```python
from build123d import *

# Parameters (mm, degrees)
F0_W     = 220
F0_H     = 25
F1_DEPTH = 15
F2_W     = 5
F2_H     = 25
F3_DEPTH = 225
F5_DEPTH = 25
F6_W     = 72.1634626389
F6_H     = 8
F7_DEPTH = 256


with BuildPart() as f1:
    # F0 (on Front) → F1 (new body)
    with BuildSketch(Plane.XZ):
        Rectangle(F0_W, F0_H)
        with BuildLine():
            Line((-62.5, 4), (62.5, 4))
            ThreePointArc((62.5, 4), (66.5, 0), (62.5, -4))
            Line((62.5, -4), (-62.5, -4))
            ThreePointArc((-62.5, -4), (-66.5, 0), (-62.5, 4))
        make_face(mode=Mode.SUBTRACT)
    extrude(amount=F1_DEPTH)

    # F2 (on face) → F3 (join)
    with BuildSketch(Plane.XZ.offset(15)):
        with Locations((-107.5, 0)):
            Rectangle(F2_W, F2_H)
        with Locations((107.5, 0)):
            Rectangle(F2_W, F2_H)
    extrude(amount=F3_DEPTH)

    # F4 (on face) → F5 (join)
    with BuildSketch(Plane(origin=(0, 0, -12.5), x_dir=(1, 0, 0), z_dir=(0, 0, -1))):
        Polygon((-110, 0), (-65, 0), (-110, 50), align=None)
        Polygon((65, 0), (110, 0), (110, 50), align=None)
    extrude(amount=-F5_DEPTH)

    # F6 (on face) → F7 (cut)
    with BuildSketch(Plane(origin=(-110, 0, 0), x_dir=(0, -1, 0), z_dir=(-1, 0, 0))):
        with Locations((186.076104641, 0)):
            Rectangle(F6_W, F6_H)
        with Locations((113.9126420021, 0)):
            Rectangle(F6_W, F6_H)
        with BuildLine():
            ThreePointArc((222.1578359604, -4), (226.1578359604, 0), (222.1578359604, 4))
            Line((222.1578359604, 4), (222.1578359604, -4))
        make_face()
        with BuildLine():
            Line((77.8309106827, -4), (77.8309106827, 4))
            ThreePointArc((77.8309106827, 4), (73.8309106827, 0), (77.8309106827, -4))
        make_face()
    extrude(amount=-F7_DEPTH, mode=Mode.SUBTRACT)


solid = f1.part
```
For this review, take the finished solid that the model builds, in its own axes (mm). A direction names the side the tool comes from. Coordinates: 2 decimals unless noted, no trailing zeros. Write each loop counter-clockwise with the first axis right and the second up, starting at its lowest first coordinate (ties: lowest second). Pieces come first, ordered by that corner, then holes.
(1) Add section D-D on x = -90. Give the boundary of the cut face in (y, z).
(2) Add section C-C on x = -17.5. Give the boundary of the cut face in (y, z), then the cut area to 3 significant figures.
(3) Add section B-B on y = -219. Give the boundary of the cut face in (x, z), then the cut area to 3 significant figures.
(4) Add section A-A on z = 0. Give the boundary of the cut face in (x, y), then the cut area to 3 significant figures.
(5) The part is to be moulded in two halves that separate along Y. For faces 1 (the face through (-108, -240, 0)), 2 (the face through (-9, -13, 12.5)), 3 (the face through (-108, -151, 4)), 4 (the face through (107.46, -73.83, 0.09)), say which applies: +Y half, -Y half, draft (parallel to the pull), parting line (faces both ways), or undercut.
(6) Tool access review of faces 5 (the face through (110, -118, -6)), 6 (the face through (1, -7, -4)), 7 (the face through (-108, -149, -4)), 8 (the face through (-66.5, -7.4, -0.1)), 9 (the face through (-1, -15, 6)): name each direction out of +Z, -Z, +X, -X, +Y, -Y from which nothing blocks a thin tool from reaching the whole face with its end or side.
(7) For pin 1 Ø1.5 at (x, z) = (17, 9) entering from -Y; pin 2 Ø6 at (x, z) = (76, 7.5) entering from -Y, all flat-tipped, find the tip position at first contact; note any pin that passes through.
(8) Wall thickness on probe 1 along X at (y, z) = (-221.5, -9.25); probe 2 along Y at (x, z) = (0, -6.25); probe 3 along X at (y, z) = (-30.5, 0): over which ranges is each line inside the solid? List them lowest first.
Answer sheet:
1. outline: (-27.78, -12.5) - (0, -12.5) - (0, 12.5) - (-27.78, 12.5) - close
2. outline: (-15, -12.5) - (0, -12.5) - (0, -4) - (-15, -4) - close; (-15, 4) - (0, 4) - (0, 12.5) - (-15, 12.5) - close
2. area: 255 mm2
3. outline: (-110, -12.5) - (-105, -12.5) - (-105, -4) - (-110, -4) - close; (-110, 4) - (-105, 4) - (-105, 12.5) - (-110, 12.5) - close; (105, -12.5) - (110, -12.5) - (110, -4) - (105, -4) - close; (105, 4) - (110, 4) - (110, 12.5) - (105, 12.5) - close
3. area: 170 mm2
4. outline: (-110, -240) - (-105, -240) - (-105, -226.16) - (-110, -226.16) - close; (-110, -73.83) - (-105, -73.83) - (-105, -44.44) - (-78.5, -15) - (-66.5, -15) - (-66.5, -1.67) - (-65, 0) - (-110, 0) - close; (65, 0) - (66.5, -1.67) - (66.5, -15) - (78.5, -15) - (105, -44.44) - (105, -73.83) - (110, -73.83) - (110, 0) - close; (105, -240) - (110, -240) - (110, -226.16) - (105, -226.16) - close
4. area: 2,810 mm2
5. face 1: -Y half
5. face 2: draft
5. face 3: undercut
5. face 4: undercut
6. face 5: +Z, -Z, +X, +Y, -Y
6. face 6: +Y, -Y
6. face 7: +X, -X
6. face 8: -Y
6. face 9: +Z, -Z, -Y
7. pin 1: stops at y = -15
7. pin 2: stops at y = -15.56
8. probe 1: x = -110 to -105, 105 to 110
8. probe 2: y = -15 to 0
8. probe 3: x = -110 to -92.45, 92.45 to 110
